from build123d import *

# Parameters (mm, degrees)
BOSS_EXTRUDE1_DEPTH        = 9.525
BOSS_EXTRUDE2_DEPTH        = 12.7
CUT_EXTRUDE1_DEPTH         = 5.08
F_10_32_TAPPED_HOLE1_D     = 4.0386
F_10_32_TAPPED_HOLE1_DEPTH = 4.445
F_10_CLEARANCE_HOLE1_D     = 4.9784
F_10_CLEARANCE_HOLE1_DEPTH = 14.604
CUT_EXTRUDE2_DEPTH         = 1.778
F_10_CLEARANCE_HOLE2_D     = 4.9784
F_10_CLEARANCE_HOLE2_DEPTH = 8.127
F_10_32_TAPPED_HOLE2_D     = 4.0386


with BuildPart() as part:
    # Sketch1 → Boss-Extrude1 (new, symmetric)
    with BuildSketch(Plane(origin=(0, 0, 0), x_dir=(1, 0, 0), z_dir=(0, 1, 0))):
        with BuildLine():
            Line((0, -6.35), (-15.875, -6.35))
            ThreePointArc((-15.875, -6.35), (-22.225, 0), (-15.875, 6.35))
            Line((-15.875, 6.35), (0, 6.35))
            Line((0, 6.35), (0, -6.35))
        make_face()
    extrude(amount=BOSS_EXTRUDE1_DEPTH, both=True)

    # Sketch2 → Boss-Extrude2 (add)
    with BuildSketch(Plane.XY.offset(6.35)):
        with BuildLine():
            Line((0, 9.525), (6.35, 9.525))
            ThreePointArc((6.35, 9.525), (15.875, 0), (6.35, -9.525))
            Line((6.35, -9.525), (0, -9.525))
            ThreePointArc((0, -9.525), (-9.525, 0), (0, 9.525))
        make_face()
    extrude(amount=-BOSS_EXTRUDE2_DEPTH)

    # Sketch3 → Cut-Extrude1 (cut, symmetric)
    with BuildSketch(Plane(origin=(0, 0, 0), x_dir=(1, 0, 0), z_dir=(0, 1, 0))):
        with BuildLine():
            Line((-9.351499966, 6.35), (-15.875, 6.35))
            ThreePointArc((-15.875, 6.35), (-22.225, 0), (-15.875, -6.35))
            Line((-15.875, -6.35), (-9.351499966, -6.35))
            Line((-9.351499966, -6.35), (-9.351499966, 6.35))
        make_face()
    extrude(amount=CUT_EXTRUDE1_DEPTH, both=True, mode=Mode.SUBTRACT)

    # #10-32 Tapped Hole1
    with Locations(Plane(origin=(0, -5.08, 0), x_dir=(1, 0, 0), z_dir=(0, 1, 0))):
        with Locations((-15.875, 0)):
            Hole(F_10_32_TAPPED_HOLE1_D / 2, depth=F_10_32_TAPPED_HOLE1_DEPTH)

    # #10 Clearance Hole1
    with Locations(Plane(origin=(0, 9.525, 0), x_dir=(1, 0, 0), z_dir=(0, 1, 0))):
        with Locations((-15.875, 0)):
            Hole(F_10_CLEARANCE_HOLE1_D / 2, depth=F_10_CLEARANCE_HOLE1_DEPTH)

    # Sketch9 → Cut-Extrude2 (cut, symmetric)
    with BuildSketch(Plane.XY):
        with BuildLine():
            Line((-3.175, 0), (-3.175, -9.525))
            Line((-3.175, -9.525), (6.35, -9.525))
            ThreePointArc((6.35, -9.525), (15.875, 0), (6.35, 9.525))
            Line((6.35, 9.525), (-3.175, 9.525))
            Line((-3.175, 9.525), (-3.175, 0))
        make_face()
    extrude(amount=CUT_EXTRUDE2_DEPTH, both=True, mode=Mode.SUBTRACT)

    # #10 Clearance Hole2
    with Locations(Plane(origin=(0, 0, -6.35), x_dir=(-1, 0, 0), z_dir=(0, 0, -1))):
        with Locations((-6.35, 0)):
            Hole(F_10_CLEARANCE_HOLE2_D / 2, depth=F_10_CLEARANCE_HOLE2_DEPTH)

    # #10-32 Tapped Hole2 (through all)
    with Locations(Plane(origin=(0, 0, 1.778), x_dir=(-1, 0, 0), z_dir=(0, 0, -1))):
        with Locations((-6.35, 0)):
            Hole(F_10_32_TAPPED_HOLE2_D / 2)


solid = part.part
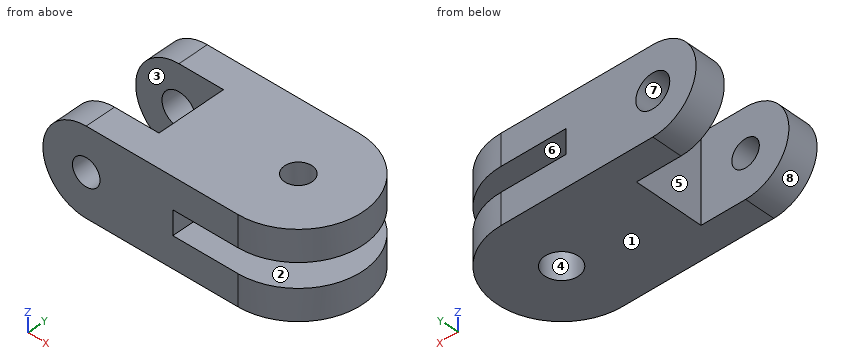
Here's how the part is built. I have some questions about the finished solid (model axes, mm). Face numbers are marked on the shaded views. A direction names the side the tool comes from. Round coordinates to 2 decimals unless told otherwise and drop trailing zeros. Order: outer loops, then holes, each group sorted by start corner. A loop starts at its lowest first (then second) coordinate and runs counter-clockwise, first axis right, second up. Notation, with made-up numbers: (28.25, -34.5) -> (63.25, -34.5) arc R18 ccw to (63.25, -18.5) -> close; hole circle Ø2 at (1, -4). An arc over 180 degrees is marked (long way). Return JSON: item names as keys, results as strings.
Q1. If we section it at C-C on y = 7.5: List the corners of the cut face in (x, z) for me (3 decimals), plus the area to 3 significant figures.
Filled sheet:
{"outline": "(-15.875, -6.35) -> (12.222, -6.35) -> (12.222, -1.778) -> (-3.175, -1.778) -> (-3.175, 1.778) -> (12.222, 1.778) -> (12.222, 6.35) -> (-15.875, 6.35) arc R6.35 ccw to start; hole circle Ø4.978 at (-15.875, 0)", "area": "346 mm^2"}
Q2. If we mould it in two halves opening along Z, with no side actions, what happens to the marked faces 1, 2 and 3? For each: released by +Z, released by -Z, zero draft, split by the parting line, or undercut.
Filled sheet:
{"face 1": "released by -Z", "face 2": "undercut", "face 3": "zero draft"}
Q3. If we section it at A-A on x = -11: List the corners of the cut face in (y, z) for me (3 decimals), plus the area to 3 significant figures.
Filled sheet:
{"outline": "(-9.525, -6.35) -> (-5.08, -6.35) -> (-5.08, 6.35) -> (-9.525, 6.35) -> close; (5.08, -6.35) -> (9.525, -6.35) -> (9.525, 6.35) -> (5.08, 6.35) -> close", "area": "113 mm^2"}
Q4. I need wall thicknesses on line 1 along Z through (x, y) = (5, -3.5); line 2 along Y through (x, z) = (-17.5, -5.25) (3 decimals); line 3 along Y through (x, z) = (6.35, 4.95) (3 decimals). Which ranges of each line are inside material? Lowest first, please. Write a range as from..to.
Filled sheet:
{"line 1": "z = -6.35..-1.78, 1.78..6.35", "line 2": "y = -9.525..-5.08, 5.08..9.525", "line 3": "y = -9.525..-2.019, 2.019..9.525"}
Q5. If we section it at B-B on z = 0: List the corners of the cut face in (x, y) for me (1 decimal).
Filled sheet:
{"outline": "(-22.2, -9.5) -> (-17.9, -9.5) -> (-17.9, -5.1) -> (-22.2, -5.1) -> close; (-22.2, 5.1) -> (-18.4, 5.1) -> (-18.4, 9.5) -> (-22.2, 9.5) -> close; (-13.9, -9.5) -> (-3.2, -9.5) -> (-3.2, 9.5) -> (-13.4, 9.5) -> (-13.4, 5.1) -> (-9.4, 5.1) -> (-9.4, -5.1) -> (-13.9, -5.1) -> close"}
Q6. For pin 1 Ø1.5 at (y, z) = (-2.5, -2) entering from +X; pin 2 Ø3 at (y, z) = (1, -3) entering from -X; pin 3 Ø1.5 at (y, z) = (-3.5, -4) entering from +X, each with a flat end and sliding along its axis, tell me the tip position at first contact or that it passes through.
Filled sheet:
{"pin 1": "stops at x = 15.71", "pin 2": "stops at x = -9.35", "pin 3": "stops at x = 15.47"}
Q7. Which directions (+Z, -Z, +X, -X, +Y, -Y) give clear straight access to the entire face, cutting with the end or side of a thin tool? Please do the marked faces 4, 5, 6, 7 and 8.
Filled sheet:
{"face 4": "-Z", "face 5": "+Z, -Z, -X", "face 6": "+X, +Y, -Y", "face 7": "+Y", "face 8": "-X, +Y, -Y"}
